Could you check a few things on this model? Use its own coordinates, in mm. A direction names the side the tool comes from. Give positions to 0.01 mm unless a question says otherwise; leave off trailing zeros. Loops run counter-clockwise (first coordinate to the right, second up) from the corner with the lowest first, then second, coordinate; pieces in that order, holes last. Notation, with made-up numbers: (-15.75, 57.5) - (9.25, 57.5) arc R26 ccw to (9.25, 82.5) - close; hole circle Ø11 at (18.5, 46). An arc over 180 degrees is marked (long way). Write each question's results on one line, items separated by ' | '. Start each with the question number.
1) I want a section at B-B, the plane z = 3.4. Count the separate pieces of the cut face and the enclosed holes in it, and give its area (3 significant figures).
2) I want a section at A-A, the plane x = -97. Write out the boundary of the cut face in (y, z).
3) If we mould it in two halves opening along X, with no side actions, what happens to faces 4 (the face through (-88.958, 0, 3)), 5 (the face through (-2.23, -123.98, 2.96)), 6 (the face through (-39, 33.75, 3))? For each: +X half, -X half, draft (parallel to the pull), parting line (faces both ways), or undercut.
4) I'm going to push flat-ended pins straight in: pin 1 (2 mm diameter, centred on x = -18.96, y = 20, fed in from -Z); pin 2 (1.8 mm diameter, centred on x = -41.5, z = 1.5, fed in from +Y) (3 decimals); pin 3 (3 mm diameter, centred on y = -95.5, z = 2, fed in from -X); pin 4 (2 mm diameter, centred on y = -69, z = 1.5, fed in from +X). Where does each tip first touch, or does it pass through?
5) I want a section at C-C, the plane y = -8.5. Write out the boundary of the cut face in (x, z), and give its area (3 significant figures).
6) If I drill on probe 1 along X at (y, z) = (-75, 2.75); probe 2 along X at (y, z) = (87, 0.7); probe 3 along Y at (x, z) = (-35.5, 1.45), over which ranges is the centre line in solid material (lowest first)? Write a range as [from, to].
7) On a 3-axis mill with a long thin cutter (end or side, diameter ignored), from which of +Z, -Z, +X, -X, +Y, -Y can I reach the whole of each face in a straight line? I mean faces 1 (the face through (-104, 35, 3)), 2 (the face through (104, -35, 3)), 3 (the face through (-20.65, -94, 3)). Say none if no direction works.
8) I want a section at D-D, the plane x = 81. Write out the boundary of the cut face in (y, z).
from build123d import *

# Parameters (mm, degrees)
ESQUISSE1_R             = 124
BOSS_EXTRU_1_DEPTH      = 6
ENL_V_MAT_EXTRU_1_DEPTH = 176.465096244
ESQUISSE3_R             = 1.65
ENL_V_MAT_EXTRU_3_DEPTH = 172.938942651
ESQUISSE5_R             = 1.65
ENL_V_MAT_EXTRU_4_DEPTH = 172.938942651
ENL_V_MAT_EXTRU_5_DEPTH = 172.938942651
ENL_V_MAT_EXTRU_6_DEPTH = 172.938942651


with BuildPart() as part:
    # Esquisse1 → Boss.-Extru.1 (new body)
    with BuildSketch(Plane.XY):
        Circle(ESQUISSE1_R)
    extrude(amount=BOSS_EXTRU_1_DEPTH)

    # Esquisse2 → Enlèv. mat.-Extru.1 (cut, through all)
    with BuildSketch(Plane.XY.offset(6)):
        with BuildLine():
            Line((-118.957975773, 35), (-88.957975773, 35))
            Line((-88.957975773, 35), (-88.957975773, -35))
            Line((-88.957975773, -35), (-118.957975773, -35))
            ThreePointArc((-118.957975773, -35), (-124, 0), (-118.957975773, 35))
        make_face()
        with BuildLine():
            Line((118.957975773, 35), (88.957975773, 35))
            Line((88.957975773, 35), (88.957975773, -35))
            Line((88.957975773, -35), (118.957975773, -35))
            ThreePointArc((118.957975773, -35), (124, 0), (118.957975773, 35))
        make_face()
    extrude(amount=-ENL_V_MAT_EXTRU_1_DEPTH, mode=Mode.SUBTRACT)

    # Esquisse3 → Enlèv. mat.-Extru.3 (cut, through all)
    with BuildSketch(Plane.XY.offset(6)):
        with Locations((-58.957975773, 20)):
            Circle(ESQUISSE3_R)
        with Locations((-18.957975773, 20)):
            Circle(ESQUISSE3_R)
        with Locations((-18.957975773, -20)):
            Circle(ESQUISSE3_R)
        with Locations((-58.957975773, -20)):
            Circle(ESQUISSE3_R)
    enl_v_mat_extru_3 = extrude(amount=-ENL_V_MAT_EXTRU_3_DEPTH, mode=Mode.SUBTRACT)

    # Esquisse5 → Enlèv. mat.-Extru.4 (cut, through all)
    with BuildSketch(Plane.XY.offset(6)):
        with Locations((-67.457975773, 45)):
            Circle(ESQUISSE5_R)
        with Locations((-67.457975773, -45)):
            Circle(ESQUISSE5_R)
    enl_v_mat_extru_4 = extrude(amount=-ENL_V_MAT_EXTRU_4_DEPTH, mode=Mode.SUBTRACT)

    # Esquisse6 → Enlèv. mat.-Extru.5 (cut, through all)
    with BuildSketch(Plane.XY.offset(6)):
        with BuildLine():
            Line((-43.957975773, 33.75), (-33.957975773, 33.75))
            ThreePointArc((-33.957975773, 33.75), (-32.707975773, 32.5), (-33.957975773, 31.25))
            Line((-33.957975773, 31.25), (-43.957975773, 31.25))
            ThreePointArc((-43.957975773, 31.25), (-45.207975773, 32.5), (-43.957975773, 33.75))
        make_face()
        with BuildLine():
            Line((-43.957975773, -31.25), (-33.957975773, -31.25))
            ThreePointArc((-33.957975773, -31.25), (-32.707975773, -32.5), (-33.957975773, -33.75))
            Line((-33.957975773, -33.75), (-43.957975773, -33.75))
            ThreePointArc((-43.957975773, -33.75), (-45.207975773, -32.5), (-43.957975773, -31.25))
        make_face()
    enl_v_mat_extru_5 = extrude(amount=-ENL_V_MAT_EXTRU_5_DEPTH, mode=Mode.SUBTRACT)

    # Esquisse7 → Enlèv. mat.-Extru.6 (cut, through all)
    with BuildSketch(Plane.XY.offset(6)):
        with BuildLine():
            Line((-17.35, 114), (-17.35, 74))
            ThreePointArc((-17.35, 74), (-19, 72.35), (-20.65, 74))
            Line((-20.65, 74), (-20.65, 114))
            ThreePointArc((-20.65, 114), (-19, 115.65), (-17.35, 114))
        make_face()
        with BuildLine():
            Line((-17.35, -74), (-17.35, -114))
            ThreePointArc((-17.35, -114), (-19, -115.65), (-20.65, -114))
            Line((-20.65, -114), (-20.65, -74))
            ThreePointArc((-20.65, -74), (-19, -72.35), (-17.35, -74))
        make_face()
    enl_v_mat_extru_6 = extrude(amount=-ENL_V_MAT_EXTRU_6_DEPTH, mode=Mode.SUBTRACT)

    # Symétrie2: Enlèv. mat.-Extru.3, Enlèv. mat.-Extru.4, Enlèv. mat.-Extru.5, Enlèv. mat.-Extru.6 across plane
    add(enl_v_mat_extru_3.mirror(Plane(origin=(0, 0, 0), x_dir=(0, 0, 1), z_dir=(1, 0, 0))), mode=Mode.SUBTRACT)
    add(enl_v_mat_extru_4.mirror(Plane(origin=(0, 0, 0), x_dir=(0, 0, 1), z_dir=(1, 0, 0))), mode=Mode.SUBTRACT)
    add(enl_v_mat_extru_5.mirror(Plane(origin=(0, 0, 0), x_dir=(0, 0, 1), z_dir=(1, 0, 0))), mode=Mode.SUBTRACT)
    add(enl_v_mat_extru_6.mirror(Plane(origin=(0, 0, 0), x_dir=(0, 0, 1), z_dir=(1, 0, 0))), mode=Mode.SUBTRACT)


solid = part.part
Answers:
1) separate pieces: 1 | enclosed holes: 20 | area: 42,800 mm2
2) outline: (-77.25, 0) - (-35, 0) - (-35, 6) - (-77.25, 6) - close; (35, 0) - (77.25, 0) - (77.25, 6) - (35, 6) - close
3) face 4: -X half | face 5: parting line | face 6: undercut
4) pin 1: passes through | pin 2: stops at y = 117.165 | pin 3: stops at x = -80.87 | pin 4: stops at x = 103.69
5) outline: (-88.96, 0) - (88.96, 0) - (88.96, 6) - (-88.96, 6) - close | area: 1,070 mm2
6) probe 1: x = [-98.75, -20.65], [-17.35, 17.35], [20.65, 98.75] | probe 2: x = [-88.36, -20.65], [-17.35, 17.35], [20.65, 88.36] | probe 3: y = [-118.81, -33.75], [-31.25, 31.25], [33.75, 118.81]
7) face 1: +Z, -Z, -X | face 2: +Z, -Z, +X | face 3: +Z, -Z
8) outline: (-93.89, 0) - (93.89, 0) - (93.89, 6) - (-93.89, 6) - close
